The listing builds one solid part. Answer for the finished solid, in the listing's coordinates (mm). Face numbers are marked on the shaded views. A direction names the side the tool comes from. Give positions to 0.01 mm unless a question says otherwise; leave off trailing zeros. Write each loop counter-clockwise with the first axis right and the second up, starting at its lowest first coordinate (ties: lowest second). Pieces come first, ordered by that corner, then holes. Notation, with made-up numbers: (60, 12.25) - (67, 12.25) arc R17 ccw to (67, 28.25) - close; hole circle Ø7 at (89, -37). An arc over 180 degrees is marked (long way). One line per question, with ' | ' between items. Start each with the question number.
1. For the marked faces 1 and 2, determine the directions among +Z, -Z, +X, -X, +Y, -Y from which every point of the face is accessible in a straight line to the end or side of a thin tool.
2. A cutting plane is placed at B-B (x = 10). Determine the outline of the cut face in (y, z), then the cut area to 3 significant figures.
3. A cutting plane is placed at D-D (y = 28). Determine the outline of the cut face in (x, z), then the cut area to 3 significant figures.
4. A cutting plane is placed at C-C (z = -3.5). Determine the outline of the cut face in (x, y), then the cut area to 3 significant figures.
5. Find the intervals of material crossed by L1, parallel to Y at x = 10, z = -3.5; L2, parallel to Y at x = 11, z = -8.5; L3, parallel to X at y = 80, z = -6.25, in increasing order. Write a range as from..to.
6. Given P1, Ø4, axis at x = 5, z = -8.66, coming from the -Y side; P2, Ø6, axis at y = 57.5, z = -3, coming from the -X side; P3, Ø4, axis at x = 10, y = 80, coming from the -Z side, each flat-ended and moving along its own axis, determine where each tip first touches the part or whether it passes through.
7. A cutting plane is placed at A-A (y = 80). Determine the outline of the cut face in (x, z).
```python
from build123d import *

# Parameters (mm, degrees)
BOSS_EXTRUDE1_DEPTH       = 85
SKETCH3_W                 = 10
SKETCH3_H                 = 2
CUT_EXTRUDE1_DEPTH        = 88.633826232
M5X0_8_TAPPED_HOLE1_D     = 4.2
M5X0_8_TAPPED_HOLE1_DEPTH = 16
M5X0_8_TAPPED_HOLE1_TIP   = 1.2618073
M5X0_8_TAPPED_HOLE2_D     = 4.2
M5X0_8_TAPPED_HOLE2_DEPTH = 16.4
M5X0_8_TAPPED_HOLE2_TIP   = 1.2618073
M3X0_5_TAPPED_HOLE1_D     = 2.5
M3X0_5_TAPPED_HOLE2_D     = 2.5


with BuildPart() as part:
    # Sketch1 → Boss-Extrude1 (new body)
    with BuildSketch(Plane(origin=(0, 0, 0), x_dir=(1, 0, 0), z_dir=(0, 1, 0))):
        Polygon((0, 0), (15, 0), (15, 4.330127019), (8.5, 14.722431864), (-3.75, 15.155444566), (-7.5, 12.990381057), align=None)
    extrude(amount=BOSS_EXTRUDE1_DEPTH)

    # Sketch3 → Cut-Extrude1 (cut, through all)
    with BuildSketch(Plane(origin=(0, 85, 0), x_dir=(1, 0, 0), z_dir=(0, 1, 0))):
        Polygon((-7.5, 12.990381057), (-5.767949192, 13.990381057), (-0.767949192, 5.330127019), (-2.5, 4.330127019), align=None)
        with Locations((10, 1)):
            Rectangle(SKETCH3_W, SKETCH3_H)
    extrude(amount=-CUT_EXTRUDE1_DEPTH, mode=Mode.SUBTRACT)

    # M5x0.8 Tapped Hole1
    with Locations(Plane(origin=(0, 85, 0), x_dir=(1, 0, 0), z_dir=(0, 1, 0))):
        with Locations((5, 8.660254038)):
            Hole(M5X0_8_TAPPED_HOLE1_D / 2, depth=M5X0_8_TAPPED_HOLE1_DEPTH)
            with Locations((0, 0, -(M5X0_8_TAPPED_HOLE1_DEPTH + M5X0_8_TAPPED_HOLE1_TIP / 2))):  # 118° drill point
                Cone(0, M5X0_8_TAPPED_HOLE1_D / 2, M5X0_8_TAPPED_HOLE1_TIP, mode=Mode.SUBTRACT)

    # M5x0.8 Tapped Hole2
    with Locations(Plane(origin=(0, 0, 0), x_dir=(-1, 0, 0), z_dir=(0, -1, 0))):
        with Locations((-5, 8.660254038)):
            Hole(M5X0_8_TAPPED_HOLE2_D / 2, depth=M5X0_8_TAPPED_HOLE2_DEPTH)
            with Locations((0, 0, -(M5X0_8_TAPPED_HOLE2_DEPTH + M5X0_8_TAPPED_HOLE2_TIP / 2))):  # 118° drill point
                Cone(0, M5X0_8_TAPPED_HOLE2_D / 2, M5X0_8_TAPPED_HOLE2_TIP, mode=Mode.SUBTRACT)

    # M3x0.5 Tapped Hole1 (through all)
    with Locations(Plane(origin=(1.732050808, 0, -1), x_dir=(0.49999999999999983, 0, 0.8660254037844387), z_dir=(-0.8660254037844387, 0, 0.49999999999999983))):
        with Locations((-10, 80), (-10, 5)):
            Hole(M3X0_5_TAPPED_HOLE1_D / 2)

    # M3x0.5 Tapped Hole2 (through all)
    with Locations(Plane.XY.offset(-2)):
        with Locations((10, 80), (10, 5)):
            Hole(M3X0_5_TAPPED_HOLE2_D / 2)


solid = part.part
```
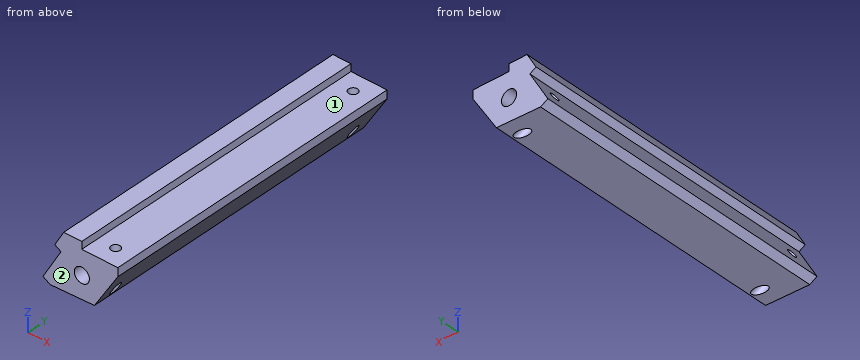
Determined:
1) face 1: +Z, +X, +Y, -Y | face 2: +Z, -Z, +X, -X, -Y
2) outline: (0, -12.32) - (3.75, -12.32) - (3.75, -2) - (0, -2) - close; (6.25, -12.32) - (78.75, -12.32) - (78.75, -2) - (6.25, -2) - close; (81.25, -12.32) - (85, -12.32) - (85, -2) - (81.25, -2) - close | area: 826 mm2
3) outline: (-5.77, -13.99) - (-3.75, -15.16) - (8.5, -14.72) - (15, -4.33) - (15, -2) - (5, -2) - (5, 0) - (0, 0) - (-2.5, -4.33) - (-0.77, -5.33) - close | area: 209 mm2
4) outline: (-2.02, 0) - (15, 0) - (15, 85) - (-2.02, 85) - close; hole circle Ø2.5 at (10, 5); hole circle Ø2.5 at (10, 80) | area: 1,440 mm2
5) L1: 0..3.75, 6.25..78.75, 81.25..85 | L2: 0..4.25, 5.75..79.25, 80.75..85 | L3: -1.3..8.75, 11.25..13.8
6) P1: y = 16.46 | P2: x = -2.5 | P3: z = -14.74
7) outline: (-5.77, -13.99) - (-3.75, -15.16) - (3.32, -14.91) - (-3.89, -10.74) - close; (-2.64, -8.58) - (8.03, -14.74) - (8.5, -14.72) - (8.75, -14.32) - (8.75, -2) - (5, -2) - (5, 0) - (0, 0) - (-2.5, -4.33) - (-0.77, -5.33) - close; (11.25, -10.33) - (15, -4.33) - (15, -2) - (11.25, -2) - close; hole circle Ø4.2 at (5, -8.66)
